Here's how the part is built. I have some questions about the finished solid (model axes, mm). A direction names the side the tool comes from. Coordinates: 2 decimals unless noted, no trailing zeros. Write each loop counter-clockwise with the first axis right and the second up, starting at its lowest first coordinate (ties: lowest second). Pieces come first, ordered by that corner, then holes.
(1) Imagine slicing it at D-D, the plane y = -3.75. List the corners of the cut face in (x, z) for me, plus the area to 3 significant figures.
(2) Please list where these lines run through material, in increasing order: probe 1 along X at (y, z) = (0, 1) (3 decimals); probe 2 along X at (y, z) = (0, 3.1) (3 decimals); probe 3 along Y at (x, z) = (-10.16, 5.6).
(3) Imagine slicing it at C-C, the plane x = 7.62. List the corners of the cut face in (y, z) for me (3 decimals).
(4) For pin 1 Ø4.5 at (x, y) = (18.415, 0) entering from +Z; pin 2 Ø7 at (x, y) = (18, 0) entering from -Z; pin 3 Ø5.5 at (x, y) = (-30, -1.5) entering from -Z; pin 4 Ø11.5 at (x, y) = (7.62, 0) entering from -Z, each with a flat end and sliding along its axis, tell me the tip position at first contact or that it passes through.
(5) Imagine slicing it at B-B, the plane y = 0. State how many separate pieces and enclosed holes the cut face has, plus the area to 3 significant figures.
(6) Imagine slicing it at A-A, the plane x = -10.16. List the corners of the cut face in (y, z) for me, plus the area to 3 significant figures.
(7) Thinking about a two-plate mould opening in Y: for faces 1 (the cylindrical face through (4.09, 2.7, 1)), 2 (the flat face through (-15, -10.16, 5)), 3 (the flat face through (0, 0, 7)), 4 (the flat face through (-15, 10.16, 5)), which applies, released by +Y, released by -Y, zero draft, split by the parting line, or undercut?
(8) Which directions (+Z, -Z, +X, -X, +Y, -Y) give clear straight access to the entire face, cutting with the end or side of a thin tool? Please do faces 5 (the flat face through (13, 0, 4.572)), 6 (the flat face through (-40.64, 0, 5)), 7 (the flat face through (20.33, 1.91, 2.032)).
```python
from build123d import *

# Parameters (mm, degrees)
F0_W          = 40.64
F0_H          = 20.32
F0_R          = 2.54
F1_DEPTH      = 9.144
F2_W          = 25.4
F2_H          = 20.32
F2_R          = 2.54
F3_DEPTH      = 4.572
F4_R          = 5.334
F4_R_2        = 2.54
F5_DEPTH      = 4.1148
F6_R          = 4.445
F6_R_2        = 2.54
F7_DEPTH      = 2.032
F8_R          = 1.5748
F9_F1_R       = 0.8128
F9_F2_R       = 0.8128
F10_T1_DEPTH  = 38.2524
F10_T3_DEPTH  = 62.8904
F10_T5_DEPTH  = 17.1704
F10_S9_W      = 0.8128
F10_S9_H      = 0.8128
F10_T10_DEPTH = 0.8128
F10_S15_W     = 0.8128
F10_S15_H     = 0.8128
F10_T16_DEPTH = 0.8128
F10_T20_ANGLE = 90
F10_T22_ANGLE = 90
F10_T24_ANGLE = 90
F10_T26_ANGLE = 90
F10_T28_ANGLE = 90
F10_T30_ANGLE = 90


# Not quite as in the source:
# - a fillet or chamfer that OpenCascade refuses, or shapes differently, is made with other operations: its cross-section is extruded or revolved along the edge and cut away or added


with BuildPart() as f1:
    # F0 (on Top) → F1 (new body)
    with BuildSketch(Plane.XY):
        with Locations((-20.32, 0)):
            Rectangle(F0_W, F0_H)
        with Locations((-29.337, 0)):
            Circle(F0_R, mode=Mode.SUBTRACT)
        with Locations((-10.16, 0)):
            Circle(F0_R, mode=Mode.SUBTRACT)
    extrude(amount=F1_DEPTH)

    # F2 (on Top) → F3 (join)
    with BuildSketch(Plane.XY):
        with Locations((12.7, 0)):
            Rectangle(F2_W, F2_H)
        with Locations((7.62, 0)):
            Circle(F2_R, mode=Mode.SUBTRACT)
        with Locations((18.415, 0)):
            Circle(F2_R, mode=Mode.SUBTRACT)
    extrude(amount=F3_DEPTH)

    # F4 (on face) → F5 (cut)
    with BuildSketch(Plane(origin=(0, 0, 0), x_dir=(1, 0, 0), z_dir=(0, 0, -1))):
        with Locations((-29.337, 0)):
            Circle(F4_R)
        with Locations((-29.337, 0)):
            Circle(F4_R_2, mode=Mode.SUBTRACT)
        with Locations((-10.16, 0)):
            Circle(F4_R)
        with Locations((-10.16, 0)):
            Circle(F4_R_2, mode=Mode.SUBTRACT)
    extrude(amount=-F5_DEPTH, mode=Mode.SUBTRACT)

    # F6 (on face) → F7 (cut)
    with BuildSketch(Plane(origin=(0, 0, 0), x_dir=(1, 0, 0), z_dir=(0, 0, -1))):
        with Locations((7.62, 0)):
            Circle(F6_R)
        with Locations((7.62, 0)):
            Circle(F6_R_2, mode=Mode.SUBTRACT)
        with Locations((18.415, 0)):
            Circle(F6_R)
        with Locations((18.415, 0)):
            Circle(F6_R_2, mode=Mode.SUBTRACT)
    extrude(amount=-F7_DEPTH, mode=Mode.SUBTRACT)

    # F8
    f8_edges = [f1.edges().sort_by_distance(p)[0] for p in [
        (-40.64, 10.16, 4.572),
        (-40.64, -10.16, 4.572),
        (25.4, 10.16, 2.286),
        (25.4, -10.16, 2.286),
    ]]
    fillet(f8_edges, radius=F8_R)

    # F9: fillet of radius 0.8128 on 3 edges, made by hand

    # F9_f1
    f9_f1_edges = [f1.edges().sort_by_distance(p)[0] for p in [
        (0, 0, 4.572),
    ]]
    fillet(f9_f1_edges, radius=F9_F1_R)

    # F9_f2
    f9_f2_edges = [f1.edges().sort_by_distance(p)[0] for p in [
        (0, 10.16, 7.2644),
        (0, 0, 9.144),
        (0.2380636083, 10.16, 4.8100636083),
    ]]
    fillet(f9_f2_edges, radius=F9_F2_R)

    # F10: fillet of radius 0.8128 on 13 edges, made by hand

    # F10_s2 → F10_t1 (cut)
    with BuildSketch(Plane.YZ.offset(-39.0652)):
        with BuildLine():
            ThreePointArc((-9.3472, 9.144), (-9.9219363917, 8.9059363917), (-10.16, 8.3312))
            Line((-10.16, 8.3312), (-10.16, 9.144))
            Line((-10.16, 9.144), (-9.3472, 9.144))
        make_face()
        with BuildLine():
            ThreePointArc((10.16, 8.3312), (9.9219363917, 8.9059363917), (9.3472, 9.144))
            Line((9.3472, 9.144), (10.16, 9.144))
            Line((10.16, 9.144), (10.16, 8.3312))
        make_face()
    extrude(amount=F10_T1_DEPTH, mode=Mode.SUBTRACT)

    # F10_s4 → F10_t3 (cut)
    with BuildSketch(Plane.YZ.offset(-39.0652)):
        with BuildLine():
            ThreePointArc((10.16, 0.8128), (9.9219363917, 0.2380636083), (9.3472, 0))
            Line((9.3472, 0), (10.16, 0))
            Line((10.16, 0), (10.16, 0.8128))
        make_face()
        with BuildLine():
            ThreePointArc((-9.3472, 0), (-9.9219363917, 0.2380636083), (-10.16, 0.8128))
            Line((-10.16, 0.8128), (-10.16, 0))
            Line((-10.16, 0), (-9.3472, 0))
        make_face()
    extrude(amount=F10_T3_DEPTH, mode=Mode.SUBTRACT)

    # F10_s6 → F10_t5 (cut)
    with BuildSketch(Plane.XZ.offset(-8.5852)):
        with BuildLine():
            ThreePointArc((-39.8272, 9.144), (-40.4019363917, 8.9059363917), (-40.64, 8.3312))
            Line((-40.64, 8.3312), (-40.64, 9.144))
            Line((-40.64, 9.144), (-39.8272, 9.144))
        make_face()
        with BuildLine():
            ThreePointArc((-39.8272, 0), (-40.4019363917, 0.2380636083), (-40.64, 0.8128))
            Line((-40.64, 0.8128), (-40.64, 0))
            Line((-40.64, 0), (-39.8272, 0))
        make_face()
        with BuildLine():
            ThreePointArc((24.5872, 0), (25.1619363917, 0.2380636083), (25.4, 0.8128))
            Line((25.4, 0.8128), (25.4, 0))
            Line((25.4, 0), (24.5872, 0))
        make_face()
    extrude(amount=F10_T5_DEPTH, mode=Mode.SUBTRACT)


with BuildPart() as f10_tool8:
    # F10_s9 → F10_t10 (new body)
    with BuildSketch(Plane.XZ.offset(-9.3472)):
        with Locations((-0.4064, 8.7376)):
            Rectangle(F10_S9_W, F10_S9_H)
    extrude(amount=-F10_T10_DEPTH)

    # F10_s11 → F10_t12 (revolve, cut)
    with BuildSketch(Plane(origin=(-0.8128, 9.3472, 8.3312), x_dir=(-0.7071067812, 0, -0.7071067812), z_dir=(0.7071067812, 0, -0.7071067812))):
        with BuildLine():
            ThreePointArc((0, -0.8128), (0.8128, 0), (0, 0.8128))
            Line((0, 0.8128), (0, -0.8128))
        make_face()
    revolve(axis=Axis((-0.8128, 9.3472, 8.3312), (0, 1, 0)), mode=Mode.SUBTRACT)


with BuildPart() as f1_1:
    add(f1.part)

    # F10_t7: cut F10_tool8
    add(f10_tool8.part, mode=Mode.SUBTRACT)


with BuildPart() as f10_tool14:
    # F10_s15 → F10_t16 (new body)
    with BuildSketch(Plane.XY.offset(8.3312)):
        with Locations((-0.4064, -9.7536)):
            Rectangle(F10_S15_W, F10_S15_H)
    extrude(amount=F10_T16_DEPTH)

    # F10_s17 → F10_t18 (revolve, cut)
    with BuildSketch(Plane(origin=(-0.8128, -9.3472, 8.3312), x_dir=(-0.7071067812, 0.7071067812, 0), z_dir=(0.7071067812, 0.7071067812, 0))):
        with BuildLine():
            ThreePointArc((0, -0.8128), (0.8128, 0), (0, 0.8128))
            Line((0, 0.8128), (0, -0.8128))
        make_face()
    revolve(axis=Axis((-0.8128, -9.3472, 8.3312), (0, 0, 1)), mode=Mode.SUBTRACT)


with BuildPart() as f1_2:
    add(f1_1.part)

    # F10_t13: cut F10_tool14
    add(f10_tool14.part, mode=Mode.SUBTRACT)

    # F10_s19 → F10_t20 (revolve, cut)
    with BuildSketch(Plane.YZ.offset(-39.0652)):
        with BuildLine():
            ThreePointArc((9.3472, 9.144), (9.9219363917, 8.9059363917), (10.16, 8.3312))
            Line((10.16, 8.3312), (10.16, 9.144))
            Line((10.16, 9.144), (9.3472, 9.144))
        make_face()
    revolve(axis=Axis((-39.0652, 8.5852, 9.144), (0, 0, 1)), revolution_arc=F10_T20_ANGLE, mode=Mode.SUBTRACT)

    # F10_s21 → F10_t22 (revolve, cut)
    with BuildSketch(Plane.XZ.offset(8.5852)):
        with BuildLine():
            ThreePointArc((-39.8272, 9.144), (-40.4019363917, 8.9059363917), (-40.64, 8.3312))
            Line((-40.64, 8.3312), (-40.64, 9.144))
            Line((-40.64, 9.144), (-39.8272, 9.144))
        make_face()
    revolve(axis=Axis((-39.0652, -8.5852, 9.144), (0, 0, 1)), revolution_arc=F10_T22_ANGLE, mode=Mode.SUBTRACT)

    # F10_s23 → F10_t24 (revolve, cut)
    with BuildSketch(Plane.YZ.offset(-39.0652)):
        with BuildLine():
            ThreePointArc((10.16, 0.8128), (9.9219363917, 0.2380636083), (9.3472, 0))
            Line((9.3472, 0), (10.16, 0))
            Line((10.16, 0), (10.16, 0.8128))
        make_face()
    revolve(axis=Axis((-39.0652, 8.5852, 0), (0, 0, 1)), revolution_arc=F10_T24_ANGLE, mode=Mode.SUBTRACT)

    # F10_s25 → F10_t26 (revolve, cut)
    with BuildSketch(Plane.XZ.offset(8.5852)):
        with BuildLine():
            ThreePointArc((-39.8272, 0), (-40.4019363917, 0.2380636083), (-40.64, 0.8128))
            Line((-40.64, 0.8128), (-40.64, 0))
            Line((-40.64, 0), (-39.8272, 0))
        make_face()
    revolve(axis=Axis((-39.0652, -8.5852, 0), (0, 0, 1)), revolution_arc=F10_T26_ANGLE, mode=Mode.SUBTRACT)

    # F10_s27 → F10_t28 (revolve, cut)
    with BuildSketch(Plane.YZ.offset(23.8252)):
        with BuildLine():
            ThreePointArc((9.3472, 0), (9.9219363917, 0.2380636083), (10.16, 0.8128))
            Line((10.16, 0.8128), (10.16, 0))
            Line((10.16, 0), (9.3472, 0))
        make_face()
    revolve(axis=Axis((23.8252, 8.5852, 0), (0, 0, -1)), revolution_arc=F10_T28_ANGLE, mode=Mode.SUBTRACT)

    # F10_s29 → F10_t30 (revolve, cut)
    with BuildSketch(Plane.XZ.offset(8.5852)):
        with BuildLine():
            ThreePointArc((24.5872, 0), (25.1619363917, 0.2380636083), (25.4, 0.8128))
            Line((25.4, 0.8128), (25.4, 0))
            Line((25.4, 0), (24.5872, 0))
        make_face()
    revolve(axis=Axis((23.8252, -8.5852, 0), (0, 0, -1)), revolution_arc=F10_T30_ANGLE, mode=Mode.SUBTRACT)


solid = f1_2.part
```
Recorded:
1. outline: (-40.64, 0.81) arc R0.81 ccw to (-39.83, 0) - (-33.13, 0) - (-33.13, 4.11) - (-25.54, 4.11) - (-25.54, 0) - (-13.95, 0) - (-13.95, 4.11) - (-6.37, 4.11) - (-6.37, 0) - (5.23, 0) - (5.23, 2.03) - (10.01, 2.03) - (10.01, 0) - (16.03, 0) - (16.03, 2.03) - (20.8, 2.03) - (20.8, 0) - (24.59, 0) arc R0.81 ccw to (25.4, 0.81) - (25.4, 3.76) arc R0.81 ccw to (24.59, 4.57) - (0.81, 4.57) arc R0.81 cw to (0, 5.38) - (0, 8.33) arc R0.81 ccw to (-0.81, 9.14) - (-39.83, 9.14) arc R0.81 ccw to (-40.64, 8.33) - close
1. area: 405 mm2
2. probe 1: x = -40.64 to -34.671, -24.003 to -15.494, -4.826 to 3.175, 12.065 to 13.97, 22.86 to 25.4
2. probe 2: x = -40.64 to -34.671, -24.003 to -15.494, -4.826 to 5.08, 10.16 to 15.875, 20.955 to 25.4
2. probe 3: y = -10.16 to -2.54, 2.54 to 10.16
3. outline: (-10.16, 0.813) arc R0.813 ccw to (-9.347, 0) - (-4.445, 0) - (-4.445, 2.032) - (-2.54, 2.032) - (-2.54, 4.572) - (-9.347, 4.572) arc R0.813 ccw to (-10.16, 3.759) - close; (2.54, 2.032) - (4.445, 2.032) - (4.445, 0) - (9.347, 0) arc R0.813 ccw to (10.16, 0.813) - (10.16, 3.759) arc R0.813 ccw to (9.347, 4.572) - (2.54, 4.572) - close
4. pin 1: passes through
4. pin 2: stops at z = 2.03
4. pin 3: stops at z = 4.11
4. pin 4: stops at z = 0
5. separate pieces: 5
5. enclosed holes: 0
5. area: 286 mm2
6. outline: (-10.16, 0.81) arc R0.81 ccw to (-9.35, 0) - (-5.33, 0) - (-5.33, 4.11) - (-2.54, 4.11) - (-2.54, 9.14) - (-9.35, 9.14) arc R0.81 ccw to (-10.16, 8.33) - close; (2.54, 4.11) - (5.33, 4.11) - (5.33, 0) - (9.35, 0) arc R0.81 ccw to (10.16, 0.81) - (10.16, 8.33) arc R0.81 ccw to (9.35, 9.14) - (2.54, 9.14) - close
6. area: 116 mm2
7. face 1: undercut
7. face 2: released by -Y
7. face 3: zero draft
7. face 4: released by +Y
8. face 5: +Z, +X, +Y, -Y
8. face 6: +Z, -Z, -X, +Y, -Y
8. face 7: -Z
